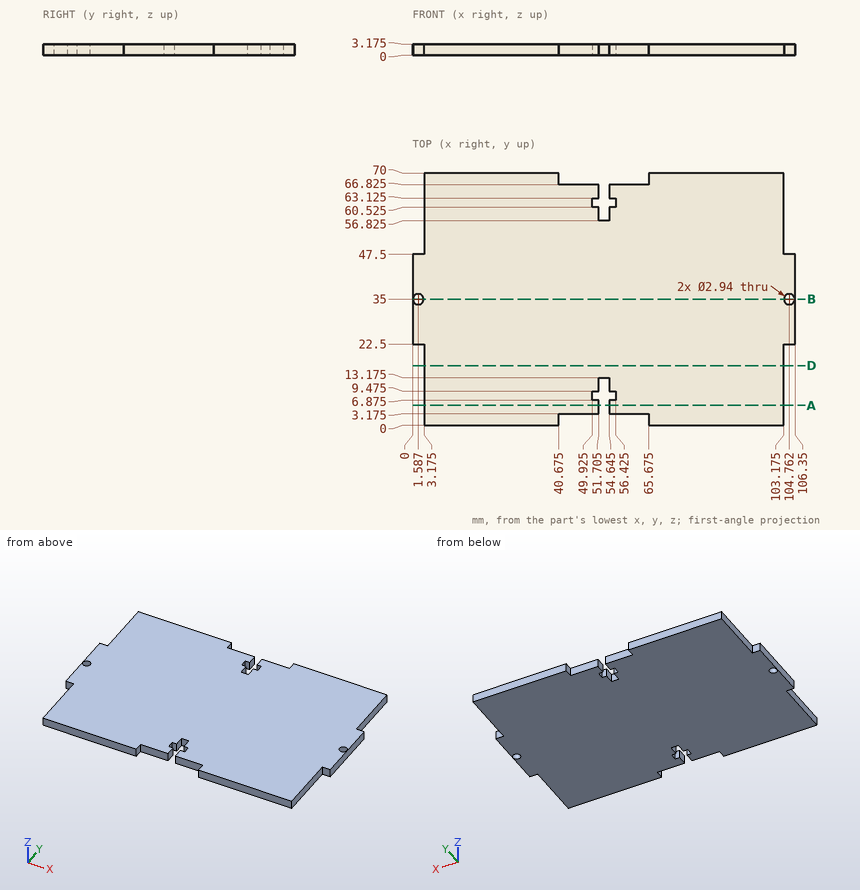
Can you work these out from the drawing? Everything is in mm from the part's minimum corner. Coordinates: 2 decimals unless noted, no trailing zeros. Write each loop counter-clockwise with the first axis right and the second up, starting at its lowest first coordinate (ties: lowest second). Pieces come first, ordered by that corner, then holes. Notation, with made-up numbers: (51, 53) - (67, 53) arc R29 ccw to (67, 82) - close; hole circle Ø9 at (65.5, 54). An arc over 180 degrees is marked (long way). Use a Markdown table: item, result.
Q1. I'm going to push flat-ended pins straight in: pin 1 Ø0.8 at (y, z) = (8, 1) entering from -X (1 decimal); pin 2 Ø1.6 at (x, z) = (1, 2) entering from +Y; pin 3 Ø1 at (y, z) = (12.5, 2) entering from +X (1 decimal); pin 4 Ø6 at (x, y) = (31.5, 36) entering from -Z. Where does each tip first touch, or does it pass through?
Geometry check:
| item | result |
|---|---|
| pin 1 | stops at x = 3.2 |
| pin 2 | stops at y = 47.5 |
| pin 3 | stops at x = 103.2 |
| pin 4 | stops at z = 0 |
Q2. Please list where these lines run through material, in increasing order: L1, parallel to Y at x = 50.5, z = 0.55 (1 decimal); L2, parallel to Y at x = 61, z = 0.45 (1 decimal); L3, parallel to X at y = 21.5, z = 1.95 (1 decimal).
Geometry check:
| item | result |
|---|---|
| L1 | y = 3.2 to 6.9, 9.5 to 60.5, 63.1 to 66.8 |
| L2 | y = 3.2 to 66.8 |
| L3 | x = 3.2 to 103.2 |
Q3. Imagine slicing it at D-D (y = 16.5). List the corners of the cut face in (x, z) for me (1 decimal).
Geometry check:
| item | result |
|---|---|
| outline | (3.2, 0) - (103.2, 0) - (103.2, 3.2) - (3.2, 3.2) - close |
Q4. Imagine slicing it at A-A (y = 5.5). List the corners of the cut face in (x, z) for me (1 decimal).
Geometry check:
| item | result |
|---|---|
| outline | (3.2, 0) - (51.7, 0) - (51.7, 3.2) - (3.2, 3.2) - close; (54.6, 0) - (103.2, 0) - (103.2, 3.2) - (54.6, 3.2) - close |
Q5. Imagine slicing it at B-B (y = 35). Count the separate pieces of the cut face and the enclosed holes in it, and give its area (3 significant figures).
Geometry check:
| item | result |
|---|---|
| separate pieces | 3 |
| enclosed holes | 0 |
| area | 319 mm2 |
